For this review, use the dimensioned drawing (mm, ordinates from the lowest corner) and the shaded views. A direction names the side the tool comes from. Give positions to 0.01 mm unless a question says otherwise; leave off trailing zeros. Write each loop counter-clockwise with the first axis right and the second up, starting at its lowest first coordinate (ties: lowest second). Pieces come first, ordered by that corner, then holes. Notation, with made-up numbers: M 23.25,27 L 39.25,27 A35 ccw 39.25,60 Z; hole C 38.25,-15 d1. An arc over 180 degrees is marked long. One line per item, written item: value. Start each with the question number.
Item 1: Consider section C-C, the plane y = 1. Write out the cut boundary in (x, z).
Item 2: Consider section A-A, the plane x = 42. Write out the cut boundary in (y, z), and give its area (3 significant figures).
Item 3: Consider section B-B, the plane y = 6.75. Write out the cut boundary in (x, z).
Item 4: Tool access review of the marked faces 4, 5 and 6: name each direction out of +Z, -Z, +X, -X, +Y, -Y from which nothing blocks a thin tool from reaching the whole face with its end or side.
Item 5: Mouldability with a two-part tool opening along Y and no side actions: class the marked faces 1, 2 and 3 as released by +Y, released by -Y, zero draft, split by the parting line, or undercut.
Item 6: Consider section D-D, the plane z = 6.5. Write out the cut boundary in (x, y), and give its area (4 significant figures).
Item 7: Clearance check with flat-ended pins moving along their axes: pin 1 Ø12 at (x, z) = (19, 5) entering from -Y; pin 2 Ø2.5 at (y, z) = (2.5, 12.5) entering from +X; pin 3 Ø3 at (x, y) = (42, 4.75) entering from -Z; pin 4 Ø1.5 at (y, z) = (2, 9) entering from -X. State where each tip first meets the part, or that it passes through.
Item 8: To check wall thickness, follow probe 1 along Y at (x, z) = (42, 2.05); probe 2 along X at (y, z) = (4.25, 1.5); probe 3 along Z at (x, y) = (7.5, 4.25). State the ranges of each line that lie inside material, in increasing order.
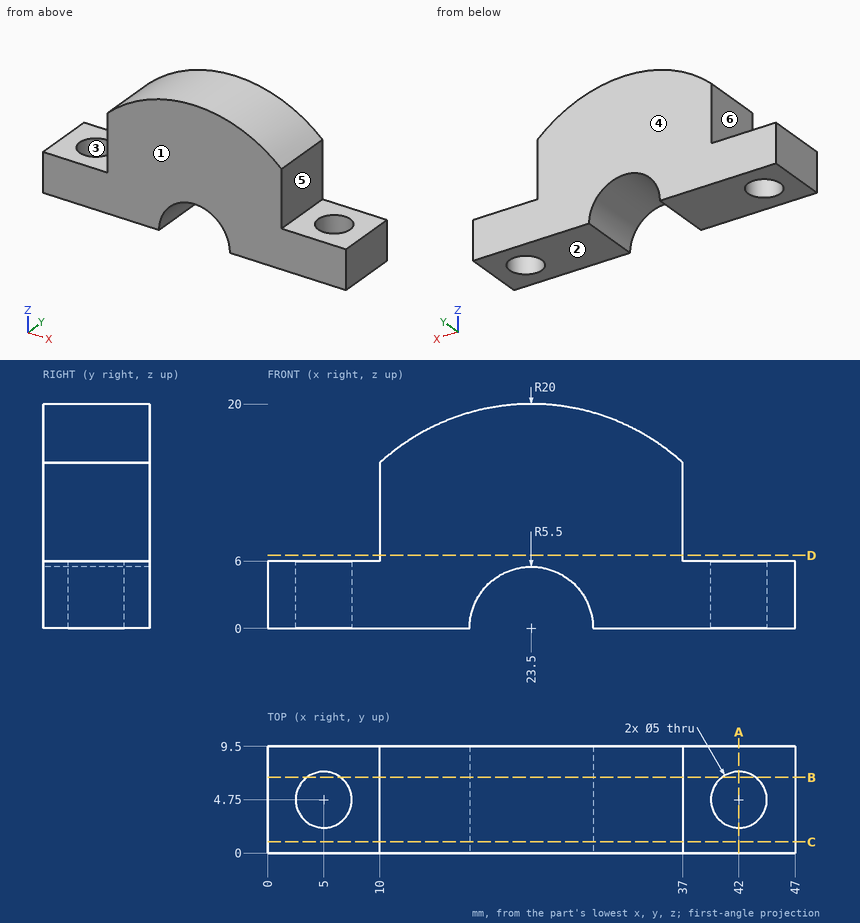
Model answer:
1. outline: M 0,0 L 18,0 A5.5 cw 29,0 L 47,0 L 47,6 L 37,6 L 37,14.76 A20 ccw 10,14.76 L 10,6 L 0,6 Z
2. outline: M 0,0 L 2.25,0 L 2.25,6 L 0,6 Z; M 7.25,0 L 9.5,0 L 9.5,6 L 7.25,6 Z
2. area: 27.0 mm2
3. outline: M 0,0 L 3.5,0 L 3.5,6 L 0,6 Z; M 6.5,0 L 18,0 A5.5 cw 29,0 L 40.5,0 L 40.5,6 L 37,6 L 37,14.76 A20 ccw 10,14.76 L 10,6 L 6.5,6 Z; M 43.5,0 L 47,0 L 47,6 L 43.5,6 Z
4. face 4: +Z, -Z, +X, -X, +Y
4. face 5: +Z, +X, +Y, -Y
4. face 6: +Z, -X, +Y, -Y
5. face 1: released by -Y
5. face 2: zero draft
5. face 3: undercut
6. outline: M 10,0 L 37,0 L 37,9.5 L 10,9.5 Z
6. area: 256.5 mm2
7. pin 1: stops at y = 0
7. pin 2: stops at x = 37
7. pin 3: passes through
7. pin 4: stops at x = 10
8. probe 1: y = 0 to 2.25, 7.25 to 9.5
8. probe 2: x = 0 to 2.55, 7.45 to 18.21, 28.79 to 39.55, 44.45 to 47
8. probe 3: z = 0 to 6
